Verification items for this drawing (mm, ordinates from the low corner). A direction names the side the tool comes from. Round coordinates to 2 decimals unless told otherwise and drop trailing zeros. Order: outer loops, then holes, each group sorted by start corner. A loop starts at its lowest first (then second) coordinate and runs counter-clockwise, first axis right, second up. Notation, with made-up numbers: M -29,69.25 L -15,69.25 A21 ccw -15,74.25 Z; hole C 19,26 d7. An arc over 180 degrees is marked long. One line per item, written item: value. Start each with the question number.
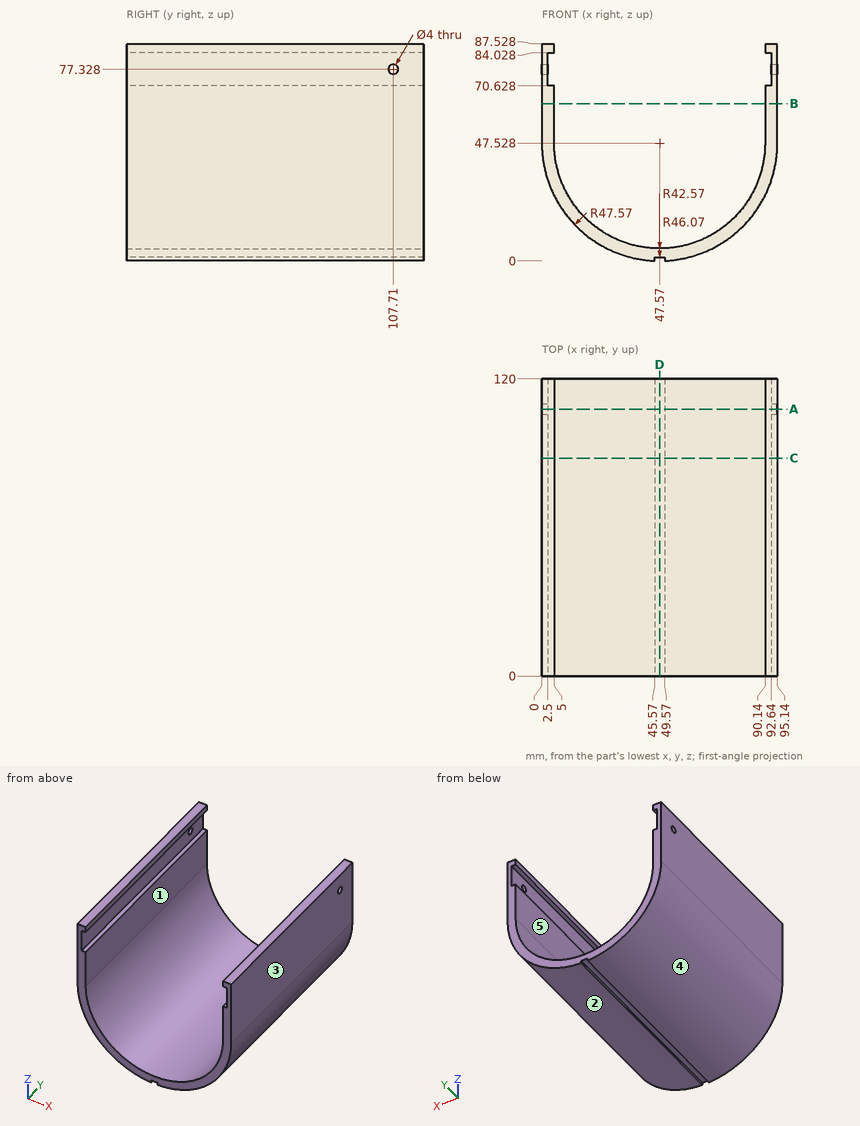
1. Section check D-D (x = 47.57). Record the cut outline in (y, z).
2. Section check A-A (y = 107.71). Record the cut outline in (x, z), and give its area (4 significant figures).
3. Section check C-C (y = 88). Record the cut outline in (x, z).
4. Scan lines: line 1 along X through (y, z) = (31, 50); line 2 along X through (y, z) = (114.5, 12.5); line 3 along Z through (x, y) = (36.5, 11.5). Record each from-to range of solid material in increasing order.
5. Draft check along X on the marked faces 3, 4 and 5. Enter one of: released by +X, released by -X, zero draft, split by the parting line, or undercut.
6. Tool access check on the marked faces 1 and 2. Record the directions out of +Z, -Z, +X, -X, +Y, -Y that give a thin tool (end or side, any length) a straight path to the whole face; none if there is none.
7. Section check B-B (z = 63.5). Record the cut outline in (x, y).
8. Depth check by flat-ended pin: pin 1 (0.8 mm diameter, centred on x = 4, y = 44.5, fed in from -Z); pin 2 (1 mm diameter, centred on x = 25.5, y = 105.5, fed in from -Z); pin 3 (1 mm diameter, centred on y = 78, z = 13.5, fed in from +X); pin 4 (3 mm diameter, centred on y = 107.71, z = 77.33, fed in from -X). Enter the tip coordinate at first touch or a pass-through.
Geometry check:
1. outline: M 0,1.46 L 120,1.46 L 120,4.96 L 0,4.96 Z
2. outline: M 0,47.53 A47.57 ccw 45.57,0 L 45.57,1.5 A46.07 ccw 49.57,1.5 L 49.57,0 A47.57 ccw 95.14,47.53 L 95.14,75.33 L 92.64,75.33 L 92.64,70.63 L 90.14,70.63 L 90.14,47.53 A42.57 cw 5,47.53 L 5,70.63 L 2.5,70.63 L 2.5,75.33 L 0,75.33 Z; M 0,79.33 L 2.5,79.33 L 2.5,84.03 L 5,84.03 L 5,87.53 L 0,87.53 Z; M 90.14,84.03 L 92.64,84.03 L 92.64,79.33 L 95.14,79.33 L 95.14,87.53 L 90.14,87.53 Z
2. area: 1,015 mm²
3. outline: M 0,47.53 A47.57 ccw 45.57,0 L 45.57,1.5 A46.07 ccw 49.57,1.5 L 49.57,0 A47.57 ccw 95.14,47.53 L 95.14,87.53 L 90.14,87.53 L 90.14,84.03 L 92.64,84.03 L 92.64,70.63 L 90.14,70.63 L 90.14,47.53 A42.57 cw 5,47.53 L 5,70.63 L 2.5,70.63 L 2.5,84.03 L 5,84.03 L 5,87.53 L 0,87.53 Z
4. line 1: x = 0 to 5, 90.14 to 95.14
4. line 2: x = 15.38 to 23.38, 71.76 to 79.76
4. line 3: z = 1.26 to 6.42
5. face 3: released by +X
5. face 4: released by -X
5. face 5: undercut
6. face 1: +Z, +Y, -Y
6. face 2: -Z, +X, +Y, -Y
7. outline: M 0,0 L 5,0 L 5,120 L 0,120 Z; M 90.14,0 L 95.14,0 L 95.14,120 L 90.14,120 Z
8. pin 1: stops at z = 27.55
8. pin 2: stops at z = 5.13
8. pin 3: stops at x = 81.32
8. pin 4: passes through
